Input: part model. Units: mm. Frame: model coordinates. A direction names the side the tool comes from. Round coordinates to 2 decimals unless told otherwise and drop trailing zeros. Loops run counter-clockwise (first coordinate to the right, second up) from the corner with the lowest first, then second, coordinate; pieces in that order, holes last. Notation, with made-up numbers: (88, 51) -> (116, 51) arc R28 ccw to (116, 70) -> close; hole circle Ø8 at (-34.5, 20.25). An arc over 180 degrees is marked (long way). Answer as a JSON object with one key per item and string values.
```python
from build123d import *

# Parameters (mm, degrees)
BOSS_EXTRUDE1_DEPTH     = 10
CUT_EXTRUDE1_DEPTH      = 38.416573868
CUT_EXTRUDE1_DEPTH_BACK = 6
SKETCH3_R               = 9.5
SKETCH4_R               = 4
CUT_EXTRUDE2_DEPTH      = 10
CUT_EXTRUDE3_DEPTH      = 51.990195136
CUT_EXTRUDE3_DEPTH_BACK = 51.990195136
SKETCH5_R               = 2


with BuildPart() as part:
    # Sketch1 → Boss-Extrude1 (new body)
    with BuildSketch(Plane(origin=(0, 0, 0), x_dir=(1, 0, 0), z_dir=(0, 1, 0))):
        Polygon((-20, -20), (20, -20), (20, 11), (30, 11), (30, 20), (20, 20), (-20, 20), (-30, 20), (-30, 11), (-20, 11), align=None)
    extrude(amount=BOSS_EXTRUDE1_DEPTH)

    # Sketch3 → Cut-Extrude1 (cut, two sides: drawn at the far end of the back side and taken through both)
    with BuildSketch(Plane(origin=(0, 10, 0), x_dir=(1, 0, 0), z_dir=(0, 1, 0)).offset(-CUT_EXTRUDE1_DEPTH_BACK)):
        with Locations(Location((0, -2, 0), (0, 0, 90))):
            Circle(SKETCH3_R)
    extrude(amount=CUT_EXTRUDE1_DEPTH + CUT_EXTRUDE1_DEPTH_BACK, mode=Mode.SUBTRACT)

    # Sketch4 → Cut-Extrude2 (cut)
    with BuildSketch(Plane(origin=(0, 4, 0), x_dir=(1, 0, 0), z_dir=(0, 1, 0))):
        with Locations(Location((0, -2, 0), (0, 0, 270))):
            Circle(SKETCH4_R)
    extrude(amount=-CUT_EXTRUDE2_DEPTH, mode=Mode.SUBTRACT)

    # Sketch5 → Cut-Extrude3 (cut, two sides: drawn at the far end of the back side and taken through both)
    with BuildSketch(Plane(origin=(0, 0, -20), x_dir=(-1, 0, 0), z_dir=(0, 0, -1)).offset(-CUT_EXTRUDE3_DEPTH_BACK)):
        with Locations((-26, 5)):
            Circle(SKETCH5_R)
        with Locations((26, 5)):
            Circle(SKETCH5_R)
    extrude(amount=CUT_EXTRUDE3_DEPTH + CUT_EXTRUDE3_DEPTH_BACK, mode=Mode.SUBTRACT)


solid = part.part
```
1) Section C-C, the plane x = 26. Output: boundary loops of the cut face in (y, z), plus the area to 3 significant figures.
Output:
{"outline": "(0, -20) -> (3, -20) -> (3, -11) -> (0, -11) -> close; (7, -20) -> (10, -20) -> (10, -11) -> (7, -11) -> close", "area": "54.0 mm^2"}
2) Draft query along Y for faces 1 (the face through (0, 0, -5)), 2 (the face through (0, 5, 20)), 3 (the face through (-27.908, 5.601, -15.437)). Return one class per face: +Y half, -Y half, draft (parallel to the pull), parting line (faces both ways), or undercut.
Output:
{"face 1": "-Y half", "face 2": "draft", "face 3": "undercut"}
3) Ray query, probe 1 along Y at (x, z) = (26, -17.5); probe 2 along X at (y, z) = (5, -18); probe 3 along X at (y, z) = (5.65, 2). Return the intervals inside material, ascending.
Output:
{"probe 1": "y = 0 to 3, 7 to 10", "probe 2": "x = -30 to -28, -24 to 24, 28 to 30", "probe 3": "x = -20 to -9.5, 9.5 to 20"}
4) Section A-A, the plane y = 5. Output: boundary loops of the cut face in (x, z).
Output:
{"outline": "(-30, -20) -> (-28, -20) -> (-28, -11) -> (-30, -11) -> close; (-24, -20) -> (24, -20) -> (24, -11) -> (20, -11) -> (20, 20) -> (-20, 20) -> (-20, -11) -> (-24, -11) -> close; (28, -20) -> (30, -20) -> (30, -11) -> (28, -11) -> close; hole circle Ø19 at (0, 2)"}
5) Contact query for flat-ended pins moving along their axis: P1, Ø5, axis at x = -25, y = 3.5, coming from the +Z side; P2, Ø1.5, axis at y = 3, z = 9, coming from the -X side; P3, Ø5, axis at y = 8, z = 0, coming from the +X side. Output: stop coordinate, or through.
Output:
{"P1": "stops at z = -11", "P2": "stops at x = -20", "P3": "stops at x = 20"}
6) Section D-D, the plane z = -13.5. Output: boundary loops of the cut face in (x, y).
Output:
{"outline": "(-30, 0) -> (30, 0) -> (30, 10) -> (-30, 10) -> close; hole circle Ø4 at (-26, 5); hole circle Ø4 at (26, 5)"}
7) Reachability of faces 4 (the face through (-20, 5, 4)), 5 (the face through (-2.854, 6.958, -7.061)), 6 (the face through (23.8, 4.9, -11)), 7 (the face through (30, 5, -15)) from +Z, -Z, +X, -X, +Y, -Y: full face, straight path, thin tool, end or side. Return the list, or none.
Output:
{"face 4": "+Z, -X, +Y, -Y", "face 5": "+Y", "face 6": "+Z, +X, +Y, -Y", "face 7": "+Z, -Z, +X, +Y, -Y"}
8) Section B-B, the plane z = 2. Output: boundary loops of the cut face in (x, y), plus the area to 3 significant figures.
Output:
{"outline": "(-20, 0) -> (-4, 0) -> (-4, 4) -> (-9.5, 4) -> (-9.5, 10) -> (-20, 10) -> close; (4, 0) -> (20, 0) -> (20, 10) -> (9.5, 10) -> (9.5, 4) -> (4, 4) -> close", "area": "254 mm^2"}
